```python
from build123d import *

# Parameters (mm, degrees)
SKETCH_1_W             = 21
SKETCH_1_H             = 0.5
EXTRUDE_1_DEPTH        = 0.4
PATTERN_LINEAR_1_COUNT = 6
PATTERN_LINEAR_1_PITCH = 3
EXTRUDE_3_DEPTH        = 0.4
PATTERN_LINEAR_2_COUNT = 8
PATTERN_LINEAR_2_PITCH = 3


with BuildPart() as part:
    # Sketch 1 → Extrude 1 (new body)
    with BuildSketch(Plane.XY):
        with Locations((10.5, 0.25)):
            Rectangle(SKETCH_1_W, SKETCH_1_H)
    extrude(amount=EXTRUDE_1_DEPTH)


with BuildPart() as pattern_linear_1_1:
    # Pattern Linear 1: pattern copy
    add(part.part.moved(Location(Vector(0, 1, 0) * (1 * PATTERN_LINEAR_1_PITCH))))


with BuildPart() as pattern_linear_1_2:
    # Pattern Linear 1: pattern copy
    add(part.part.moved(Location(Vector(0, 1, 0) * (2 * PATTERN_LINEAR_1_PITCH))))


with BuildPart() as pattern_linear_1_3:
    # Pattern Linear 1: pattern copy
    add(part.part.moved(Location(Vector(0, 1, 0) * (3 * PATTERN_LINEAR_1_PITCH))))


with BuildPart() as pattern_linear_1_4:
    # Pattern Linear 1: pattern copy
    add(part.part.moved(Location(Vector(0, 1, 0) * (4 * PATTERN_LINEAR_1_PITCH))))


with BuildPart() as pattern_linear_1_5:
    # Pattern Linear 1: pattern copy
    add(part.part.moved(Location(Vector(0, 1, 0) * (5 * PATTERN_LINEAR_1_PITCH))))


with BuildPart() as part_1:
    add(part.part)

    add(pattern_linear_1_1.part)  # Extrude 3 merges Pattern Linear 1_1

    add(pattern_linear_1_2.part)  # Extrude 3 merges Pattern Linear 1_2

    add(pattern_linear_1_3.part)  # Extrude 3 merges Pattern Linear 1_3
    # Sketch 3 → Extrude 3 (add)
    with BuildSketch(Plane.XY.offset(0.4)):
        Polygon((0, 15.5), (0, 9.5), (0, 0), (-0.5, 0), (-0.5, 10.98507125), (-0.5, 15.5), align=None)
    extrude_3 = extrude(amount=-EXTRUDE_3_DEPTH)

    # Pattern Linear 2: Extrude 3 ×8
    with Locations(*[(i * PATTERN_LINEAR_2_PITCH, 0, 0) for i in range(1, PATTERN_LINEAR_2_COUNT)]):
        add(extrude_3)

    # Combine 1: read off the stored shape, not the designer's step
    # Combine 1: union Pattern Linear 1_4, Pattern Linear 1_5
    add(pattern_linear_1_4.part)
    add(pattern_linear_1_5.part)


solid = part_1.part
```
Verification items for the finished model (mm, model axes). Coordinates: 2 decimals unless noted, no trailing zeros. Loops run counter-clockwise (first coordinate to the right, second up) from the corner with the lowest first, then second, coordinate; pieces in that order, holes last. Notation, with made-up numbers: (-2.75, 77) -> (51.25, 77) arc R16 ccw to (51.25, 97) -> close; hole circle Ø11 at (-1, 69.25). An arc over 180 degrees is marked (long way). Answer in a Markdown table with one row per item. Add a question column.
1. Section check B-B, the plane x = 13.75. Enter the section's corners in (y, z).
2. Section check A-A, the plane y = 1.5. Give the number of separate pieces and of enclosed holes in the cut face, then the cut area to 3 significant figures.
3. Depth check by flat-ended pin: P1, Ø5, axis at x = 4, y = 10, coming from the -Z side. Enter the tip coordinate at first touch or a pass-through.
4. Material ranges on probe 1 along Y at (x, z) = (14, 0.35), recorded low to high. Write a range as [from, to].
Derived:
| question | item | result |
|---|---|---|
| 1 | outline | (0, 0) -> (0.5, 0) -> (0.5, 0.4) -> (0, 0.4) -> close; (3, 0) -> (3.5, 0) -> (3.5, 0.4) -> (3, 0.4) -> close; (6, 0) -> (6.5, 0) -> (6.5, 0.4) -> (6, 0.4) -> close; (9, 0) -> (9.5, 0) -> (9.5, 0.4) -> (9, 0.4) -> close; (12, 0) -> (12.5, 0) -> (12.5, 0.4) -> (12, 0.4) -> close; (15, 0) -> (15.5, 0) -> (15.5, 0.4) -> (15, 0.4) -> close |
| 2 | separate pieces | 8 |
| 2 | enclosed holes | 0 |
| 2 | area | 1.60 mm² |
| 3 | P1 | stops at z = 0 |
| 4 | probe 1 | y = [0, 0.5], [3, 3.5], [6, 6.5], [9, 9.5], [12, 12.5], [15, 15.5] |
